For this review, take the finished solid that the model builds, in its own axes (mm). A direction names the side the tool comes from. Round coordinates to 2 decimals unless told otherwise and drop trailing zeros. Write each loop counter-clockwise with the first axis right and the second up, starting at its lowest first coordinate (ties: lowest second). Pieces come first, ordered by that corner, then holes. Notation, with made-up numbers: (-40, 41) -> (3, 41) arc R7 cw to (3, 46) -> close; hole circle Ø11 at (80.5, 57). An arc over 180 degrees is marked (long way). Answer as CSV lines item,"result". Start each with the question number.
Item 1: Take a section at D-D on x = 71.5. Give the boundary of the cut face in (y, z), then the cut area to 3 significant figures.
Item 2: Take a section at A-A on x = 0. Count the separate pieces of the cut face and the enclosed holes in it, then the cut area to 3 significant figures.
Item 3: Mouldability with a two-part tool opening along Y and no side actions: class faces 4 (the cylindrical face through (-84.14, -64.1, 0.04)), 5 (the flat face through (-65, -49, 5)), 6 (the flat face through (49, -11, 2)) as +Y half, -Y half, draft (parallel to the pull), parting line (faces both ways), or undercut.
Item 4: Take a section at B-B on x = -19. Give the boundary of the cut face in (y, z), then the cut area to 3 significant figures.
Item 5: For pin 1 Ø2 at (y, z) = (-27, -10) entering from -X; pin 2 Ø1 at (x, y) = (66.5, -38) entering from +Z; pin 3 Ø1 at (x, z) = (-32, -4) entering from -Y, all flat-tipped, find the tip position at first contact; note any pin that passes through.
Item 6: Take a section at C-C on y = -58. Give the boundary of the cut face in (x, z).
Item 7: Machinability: for faces 1 (the flat face through (49, -32, 0)), 2 (the flat face through (-35, -2, -13)), 3 (the flat face through (1, -32, 4.5)), which of the approach directions +Z, -Z, +X, -X, +Y, -Y give a long, thin tool a straight path to every point of the face, cutting with its end or side? Answer none if there is none.
Item 8: Wall thickness on probe 1 along X at (y, z) = (-26, -9); probe 2 along Y at (x, z) = (1, -5); probe 3 along Z at (x, y) = (0, -3.1): over which ranges is each line inside the solid? List them lowest first. Write a range as from..to.
```python
from build123d import *

# Parameters (mm, degrees)
F0_W        = 170
F0_H        = 6
F1_DEPTH    = 65
F2_W        = 48.5
F2_H        = 43
F3_DEPTH    = 3
F4_W        = 70
F4_H        = 4
F5_DEPTH    = 4
F6_W        = 69.1558677684
F6_H        = 4
F6_W_2      = 69.5469340682
F6_H_2      = 6
F7_DEPTH    = 30
F8_W        = 5
F8_H        = 30
F9_DEPTH    = 20
F10_SIZE2   = 18
F10_SIZE    = 28
F10_2_SIZE2 = 18
F10_2_SIZE  = 28
F11_W       = 14.7919125855
F11_H       = 2.5
F11_W_2     = 15.1694379747
F12_DEPTH   = 36.001
F13_R       = 10
F14_R       = 1.5
F15_R       = 1.5
F16_R       = 3
F18_DEPTH   = 119.5479340682
F20_D       = 4
F21_W       = 10
F21_H       = 25
F22_DEPTH   = 25
F23_R       = 5
F24_R       = 2
F25_R       = 2
F26_R       = 1.5
F27_W       = 8
F27_H       = 30
F28_DEPTH   = 1.5


with BuildPart() as f1:
    # F0 (on Front) → F1 (new body)
    with BuildSketch(Plane.XZ):
        Rectangle(F0_W, F0_H)
    extrude(amount=F1_DEPTH)

    # F2 (on face) → F3 (cut)
    with BuildSketch(Plane.XY.offset(3)):
        with Locations((49.75, -32.5)):
            Rectangle(F2_W, F2_H)
    extrude(amount=-F3_DEPTH, mode=Mode.SUBTRACT)

    # F4 (on face) → F5 (join)
    with BuildSketch(Plane.XY.offset(3)):
        with Locations((-30, -15)):
            Rectangle(F4_W, F4_H)
        with Locations((-30, -49)):
            Rectangle(F4_W, F4_H)
    extrude(amount=F5_DEPTH)

    # F6 (on face) → F7 (join)
    with BuildSketch(Plane(origin=(0, 0, -3), x_dir=(1, 0, 0), z_dir=(0, 0, -1))):
        with Locations((-0.030999816, 14.5)):
            Rectangle(F6_W, F6_H)
        with Locations((-0.2265329659, 3)):
            Rectangle(F6_W_2, F6_H_2)
    extrude(amount=F7_DEPTH)

    # F8 (on face) → F9 (join)
    with BuildSketch(Plane.XZ.offset(16.5)):
        with Locations((-32.1089337002, -18)):
            Rectangle(F8_W, F8_H)
        with Locations((32.0469340682, -18)):
            Rectangle(F8_W, F8_H)
    extrude(amount=F9_DEPTH)

    # F10
    f10_edges = [f1.edges().sort_by_distance(p)[0] for p in [
        (-32.108934, -36.5, -33),
    ]]
    f10_side = f1.faces().sort_by_distance((-32.108934, -36.5, -18))[0]
    chamfer(f10_edges, length=F10_SIZE, length2=F10_SIZE2, reference=f10_side)

    # F10#2
    f10_2_edges = [f1.edges().sort_by_distance(p)[0] for p in [
        (32.046934, -36.5, -33),
    ]]
    f10_2_side = f1.faces().sort_by_distance((32.046934, -36.5, -18))[0]
    chamfer(f10_2_edges, length=F10_2_SIZE, length2=F10_2_SIZE2, reference=f10_2_side)

    # F11 (on face) → F12 (cut, through all)
    with BuildSketch(Plane.XY.offset(3)):
        with Locations((-42.6040437073, -11.75)):
            Rectangle(F11_W, F11_H)
        with Locations((-42.4152810127, -52.25)):
            Rectangle(F11_W_2, F11_H)
    extrude(amount=-F12_DEPTH, mode=Mode.SUBTRACT)

    # F13
    f13_edges = [f1.edges().sort_by_distance(p)[0] for p in [
        (-35, -3, -33),
        (34.546934, -3, -33),
    ]]
    fillet(f13_edges, radius=F13_R)

    # F14
    f14_edges = [f1.edges().sort_by_distance(p)[0] for p in [
        (-34.608934, -12.5, -18),
        (34.546934, -12.5, -18),
        (-0.031, -12.5, -33),
    ]]
    fillet(f14_edges, radius=F14_R)

    # F15
    f15_edges = [f1.edges().sort_by_distance(p)[0] for p in [
        (34.546934, -6, -13),
        (31.618002, -6, -30.071068),
        (-0.226533, -6, -33),
        (-32.071068, -6, -30.071068),
        (-35, -6, -13),
    ]]
    fillet(f15_edges, radius=F15_R)

    # F16
    f16_edges = [f1.edges().sort_by_distance(p)[0] for p in [
        (-85, -65, 0),
        (-85, 0, 0),
        (85, 0, 0),
        (85, -65, 0),
    ]]
    fillet(f16_edges, radius=F16_R)

    # F17 (on face) → F18 (cut, through all)
    with BuildSketch(Plane.YZ.offset(34.5469340682)):
        with BuildLine():
            Line((-18.5, -33), (-16.25, -33))
            ThreePointArc((-16.25, -33), (-21.5712447444, -15.5258555741), (-36.5, -5))
            Line((-36.5, -5), (-18.5, -33))
        make_face()
    extrude(amount=-F18_DEPTH, mode=Mode.SUBTRACT)

    # F20 (through all)
    with Locations(Plane(origin=(0, 0, 0), x_dir=(-1, 0, 0), z_dir=(0, 1, 0))):
        with Locations((0, -12.6412017271)):
            Hole(F20_D / 2)

    # F21 (on face) → F22 (cut)
    with BuildSketch(Plane.XY.offset(3)):
        with Locations((-80, -32.5)):
            Rectangle(F21_W, F21_H)
    extrude(amount=-F22_DEPTH, mode=Mode.SUBTRACT)

    # F23
    f23_edges = [f1.edges().sort_by_distance(p)[0] for p in [
        (-75, -20, 0),
        (-75, -45, 0),
    ]]
    fillet(f23_edges, radius=F23_R)

    # F24
    f24_edges = [f1.edges().sort_by_distance(p)[0] for p in [
        (-75, -32.5, 3),
        (-76.464466, -21.464466, 3),
        (-82.5, -20, 3),
        (-76.464466, -43.535534, 3),
        (-82.5, -45, 3),
    ]]
    fillet(f24_edges, radius=F24_R)

    # F25
    f25_edges = [f1.edges().sort_by_distance(p)[0] for p in [
        (-82.5, -45, -3),
        (-76.464466, -43.535534, -3),
        (-75, -32.5, -3),
        (-76.464466, -21.464466, -3),
        (-82.5, -20, -3),
    ]]
    fillet(f25_edges, radius=F25_R)

    # F26
    f26_edges = [f1.edges().sort_by_distance(p)[0] for p in [
        (-30, -13, 7),
        (-30, -51, 7),
    ]]
    fillet(f26_edges, radius=F26_R)

    # F27 (on face) → F28 (join)
    with BuildSketch(Plane.XY.offset(3)):
        with Locations((1, -32)):
            Rectangle(F27_W, F27_H)
    extrude(amount=F28_DEPTH)


solid = f1.part
```
Output values:
1,outline,"(-65, -3) -> (0, -3) -> (0, 3) -> (-11, 3) -> (-11, 0) -> (-54, 0) -> (-54, 3) -> (-65, 3) -> close"
1,area,"261 mm^2"
2,separate pieces,"3"
2,enclosed holes,"0"
2,area,"724 mm^2"
3,face 4,"-Y half"
3,face 5,"draft"
3,face 6,"undercut"
4,outline,"(-65, -3) -> (-16.5, -3) -> (-16.5, -28.15) arc R28.14 cw to (-16.25, -33) -> (-14, -33) arc R1.5 ccw to (-12.5, -31.5) -> (-12.5, -3) -> (-6, -3) -> (-6, -31.5) arc R1.5 ccw to (-4.5, -33) -> (0, -33) -> (0, 3) -> (-13, 3) -> (-13, 5.5) arc R1.5 ccw to (-14.5, 7) -> (-17, 7) -> (-17, 3) -> (-47, 3) -> (-47, 7) -> (-49.5, 7) arc R1.5 ccw to (-51, 5.5) -> (-51, 3) -> (-65, 3) -> close"
4,area,"719 mm^2"
5,pin 1,"stops at x = -34.61"
5,pin 2,"stops at z = 0"
5,pin 3,"stops at y = -36.5"
6,outline,"(-85, -3) -> (85, -3) -> (85, 3) -> (-85, 3) -> close"
7,face 1,"+Z"
7,face 2,"-Z, -X, +Y, -Y"
7,face 3,"+Z, +X, -X"
8,probe 1,"x = -34.61..-29.61, 29.55..34.55"
8,probe 2,"y = -16.5..-12.5, -6..0"
8,probe 3,"z = -33..-14.64, -10.64..3"
